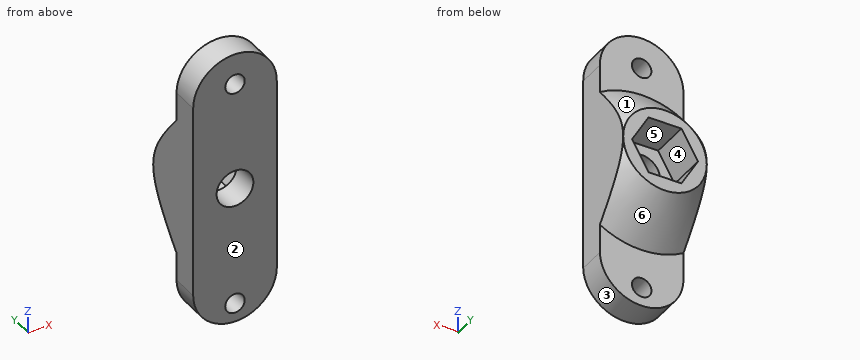
from build123d import *

# Parameters (mm, degrees)
F1_DEPTH     = 5
F2_R         = 7.5
F3_DEPTH     = 7
F5_D         = 6.6
F7_DEPTH     = 7
F9_T4_ANGLE  = 179.9999997857
F9_T10_ANGLE = 180.0000002143
F10_D        = 3.5


# Not quite as in the source:
# - a fillet or chamfer that OpenCascade refuses, or shapes differently, is made with other operations: its cross-section is extruded or revolved along the edge and cut away or added


with BuildPart() as f1:
    # F0 (on Front) → F1 (new body)
    with BuildSketch(Plane.XZ):
        with BuildLine():
            ThreePointArc((-7.5, -17.4188318139), (-0.0794529453, -24.9192617628), (7.5, -17.5794483415))
            Line((7.5, -17.5794483415), (7.5, 17.4188318139))
            ThreePointArc((7.5, 17.4188318139), (0.0811727899, 25.0798782903), (-7.5, 17.5794483415))
            Line((-7.5, 17.5794483415), (-7.5, -17.4188318139))
        make_face()
    extrude(amount=F1_DEPTH)

    # F2 (on face) → F3 (join)
    with BuildSketch(Plane(origin=(0, 0, 0), x_dir=(-1, 0, 0), z_dir=(0, 1, 0))):
        Circle(F2_R)
    extrude(amount=F3_DEPTH)

    # F5 (through all)
    with Locations(Plane.XZ.offset(5)):
        with Locations((0, 0)):
            Hole(F5_D / 2)

    # F6 (on face) → F7 (cut, through all)
    with BuildSketch(Plane(origin=(0, 7, 0), x_dir=(-1, 0, 0), z_dir=(0, 1, 0))):
        Polygon((2.9589201296, -5.125), (5.9178402592, 0), (2.9589201296, 5.125), (-2.9589201296, 5.125), (-5.9178402592, 0), (-2.9589201296, -5.125), align=None)
    extrude(amount=-F7_DEPTH, mode=Mode.SUBTRACT)

    # F9: chamfer of 7 on 2 edges, made by hand


with BuildPart() as f9_tool2:
    # F9_s3 → F9_t4 (revolve)
    with BuildSketch(Plane.XY):
        Polygon((-14.5, 0), (-7.5, 7), (-7.5, 0), align=None)
    revolve(axis=Axis((0, 0, 0), (0, 1, 0)), revolution_arc=F9_T4_ANGLE)

    split(bisect_by=Plane.YZ.offset(-7.5), keep=Keep.TOP)

    split(bisect_by=Plane.YZ.offset(7.5), keep=Keep.BOTTOM)


with BuildPart() as f1_1:
    add(f1.part)

    # F9_t1: union F9_tool2
    add(f9_tool2.part)


with BuildPart() as f9_tool8:
    # F9_s9 → F9_t10 (revolve)
    with BuildSketch(Plane.XY):
        Polygon((14.5, 0), (7.5, 7), (7.5, 0), align=None)
    revolve(axis=Axis((0, 0, 0), (0, 1, 0)), revolution_arc=F9_T10_ANGLE)

    split(bisect_by=Plane.YZ.offset(-7.5), keep=Keep.TOP)

    split(bisect_by=Plane.YZ.offset(7.5), keep=Keep.BOTTOM)


with BuildPart() as f1_2:
    add(f1_1.part)

    # F9_t7: union F9_tool8
    add(f9_tool8.part)

    # F10 (through all)
    with Locations(Plane.XZ.offset(5)):
        with Locations((0.0010000484, 19.5), (0, -21.5)):
            Hole(F10_D / 2)


solid = f1_2.part
Here's how the part is built. I have some questions about the finished solid (model axes, mm). Face numbers are marked on the shaded views. A direction names the side the tool comes from. Coordinates: 2 decimals unless noted, no trailing zeros. Write each loop counter-clockwise with the first axis right and the second up, starting at its lowest first coordinate (ties: lowest second). Pieces come first, ordered by that corner, then holes.
Item 1: If we mould it in two halves opening along Z, with no side actions, what happens to the marked faces 1, 2, 3 and 4? For each: +Z half, -Z half, draft (parallel to the pull), parting line (faces both ways), or undercut.
Item 2: I want a section at B-B on z = 19.5. Write out the boundary of the cut face in (x, y).
Item 3: I want a section at C-C on y = -2.75. Write out the boundary of the cut face in (x, z).
Item 4: Will these pins go through, and if not, where does the flat tip stop? pin 1 (1.5 mm diameter, centred on x = 2.5, z = -2, fed in from +Y); pin 2 (1.8 mm diameter, centred on x = 0, y = 4.5, fed in from -Z); pin 3 (2 mm diameter, centred on x = 3.5, y = 3, fed in from +Z).
Item 5: I want a section at A-A on x = 0. Write out the boundary of the cut face in (y, z) (3 decimals).
Item 6: I want a section at D-D on y = 3.25. Write out the boundary of the cut face in (x, z) (3 decimals), and give its area (3 significant figures).
Item 7: On a 3-axis mill with a long thin cutter (end or side, diameter ignored), from which of +Z, -Z, +X, -X, +Y, -Y can I reach the whole of each face in a straight line? I mean the marked faces 5 and 6. Say none if no direction works.
Item 8: If I drill on line 1 (Z direction, x = 0, y = -1.3); line 2 (Y direction, x = 0, z = 22); line 3 (X direction, y = 6.75, z = 3), over which ranges is the centre line in solid material (lowest first)?
Findings below:
1. face 1: +Z half
1. face 2: draft
1. face 3: -Z half
1. face 4: undercut
2. outline: (-7.25, -5) - (-1.75, -5) - (-1.75, 0) - (-7.25, 0) - close; (1.75, -5) - (7.25, -5) - (7.25, 0) - (1.75, 0) - close
3. outline: (-7.5, -17.42) arc R7.5 ccw to (7.5, -17.58) - (7.5, 17.42) arc R7.5 ccw (long way) to (-7.5, 17.58) - close; hole circle Ø6.6 at (0, 0); hole circle Ø3.5 at (0, -21.5); hole circle Ø3.5 at (0, 19.5)
4. pin 1: stops at y = 0
4. pin 2: stops at z = -10.9
4. pin 3: stops at z = 12.04
5. outline: (-5, -24.92) - (0, -24.92) - (0, -23.25) - (-5, -23.25) - close; (-5, -19.75) - (0, -19.75) - (0, -14.5) - (7, -7.5) - (7, -5.125) - (0, -5.125) - (0, -3.3) - (-5, -3.3) - close; (-5, 3.3) - (0, 3.3) - (0, 5.125) - (7, 5.125) - (7, 7.5) - (0, 14.5) - (0, 17.75) - (-5, 17.75) - close; (-5, 21.25) - (0, 21.25) - (0, 25.08) - (-5, 25.08) - close
6. outline: (-7.5, -8.385) arc R11.25 ccw to (7.5, -8.385) - (7.5, 8.385) arc R11.25 ccw to (-7.5, 8.385) - close; hole (-5.918, 0) - (-2.959, -5.125) - (2.959, -5.125) - (5.918, 0) - (2.959, 5.125) - (-2.959, 5.125) - close
6. area: 220 mm2
7. face 5: +Y
7. face 6: -Z, +Y
8. line 1: z = -24.92 to -23.25, -19.75 to -3.3, 3.3 to 17.75, 21.25 to 25.08
8. line 2: y = -5 to 0
8. line 3: x = -7.15 to -4.19, 4.19 to 7.15
